Here's how the part is built. I have some questions about the finished solid (model axes, mm). A direction names the side the tool comes from. Give positions to 0.01 mm unless a question says otherwise; leave off trailing zeros. Write each loop counter-clockwise with the first axis right and the second up, starting at its lowest first coordinate (ties: lowest second). Pieces come first, ordered by that corner, then holes. Notation, with made-up numbers: (19, 17) -> (46, 17) arc R25 ccw to (46, 56) -> close; hole circle Ø7 at (-30.5, 79). An arc over 180 degrees is marked (long way). Return JSON: item names as keys, results as strings.
from build123d import *

# Parameters (mm, degrees)
EXTRUDE_1_DEPTH     = 11
SKETCH_2_R          = 2.05
CUT_EXTRUDE_1_DEPTH = 12
SKETCH_3_R          = 3.6
CUT_EXTRUDE_2_DEPTH = 10


with BuildPart() as part:
    # 草图1 → 凸台-拉伸1 (new body)
    with BuildSketch(Plane(origin=(0, 0, 0), x_dir=(1, 0, 0), z_dir=(0, 1, 0))):
        with BuildLine():
            Line((-6, -13), (-6, 13))
            ThreePointArc((-6, 13), (0, 19), (6, 13))
            Line((6, 13), (6, -13))
            ThreePointArc((6, -13), (0, -19), (-6, -13))
        make_face()
    extrude(amount=EXTRUDE_1_DEPTH)

    # 草图2 → 切除-拉伸1 (cut, through all)
    with BuildSketch(Plane(origin=(0, 11, 0), x_dir=(1, 0, 0), z_dir=(0, 1, 0))):
        with Locations((0, 13)):
            Circle(SKETCH_2_R)
        with Locations((0, -13)):
            Circle(SKETCH_2_R)
    extrude(amount=-CUT_EXTRUDE_1_DEPTH, mode=Mode.SUBTRACT)

    # 草图3 → 切除-拉伸2 (cut)
    with BuildSketch(Plane.ZY.offset(6)):
        with Locations((0, 5.5)):
            Circle(SKETCH_3_R)
    extrude(amount=-CUT_EXTRUDE_2_DEPTH, mode=Mode.SUBTRACT)


solid = part.part
1. If I drill on line 1 (Y direction, x = 1.25, z = 0); line 2 (Z direction, x = 0.5, y = 1.75); line 3 (Z direction, x = 0, y = 3.25), over which ranges is the centre line in solid material (lowest first)? Write a range as [from, to].
Taken from the geometry:
{"line 1": "y = [0, 1.9], [9.1, 11]", "line 2": "z = [-18.98, -14.99], [-11.01, 11.01], [14.99, 18.98]", "line 3": "z = [-19, -15.05], [-10.95, -2.81], [2.81, 10.95], [15.05, 19]"}
2. Suppose I cut it at C-C, the plane z = -14. List the corners of the cut face in (x, y) for me.
Taken from the geometry:
{"outline": "(-5.92, 0) -> (-1.79, 0) -> (-1.79, 11) -> (-5.92, 11) -> close; (1.79, 0) -> (5.92, 0) -> (5.92, 11) -> (1.79, 11) -> close"}
3. Suppose I cut it at A-A, the plane x = 0. List the corners of the cut face in (y, z) for me.
Taken from the geometry:
{"outline": "(0, -19) -> (11, -19) -> (11, -15.05) -> (0, -15.05) -> close; (0, -10.95) -> (11, -10.95) -> (11, 10.95) -> (0, 10.95) -> close; (0, 15.05) -> (11, 15.05) -> (11, 19) -> (0, 19) -> close; hole circle Ø7.2 at (5.5, 0)"}
4. Suppose I cut it at D-D, the plane z = 0. List the corners of the cut face in (x, y) for me.
Taken from the geometry:
{"outline": "(-6, 0) -> (6, 0) -> (6, 11) -> (-6, 11) -> (-6, 9.1) -> (4, 9.1) -> (4, 1.9) -> (-6, 1.9) -> close"}
5. Which directions (+Z, -Z, +X, -X, +Y, -Y) give clear straight access to the entire face, cutting with the end or side of a thin tool? Please do faces 1 (the face through (-6, 3, 3)), 2 (the face through (-1.07, 9.07, -0.47)).
Taken from the geometry:
{"face 1": "+Z, -Z, -X, +Y, -Y", "face 2": "-X"}
6. Suppose I cut it at B-B, the plane y = 1. List the corners of the cut face in (x, z) for me, and give its area (3 significant figures).
Taken from the geometry:
{"outline": "(-6, -13) arc R6 ccw to (6, -13) -> (6, 13) arc R6 ccw to (-6, 13) -> close; hole circle Ø4.1 at (0, -13); hole circle Ø4.1 at (0, 13)", "area": "399 mm²"}
7. If we mould it in two halves opening along X, with no side actions, what happens to faces 3 (the face through (6, 5, 0)), 4 (the face through (-0.444, 5.577, 15.001)), 5 (the face through (0, 5, 19))? For each: released by +X, released by -X, zero draft, split by the parting line, or undercut.
Taken from the geometry:
{"face 3": "released by +X", "face 4": "undercut", "face 5": "split by the parting line"}
8. For pin 1 Ø5 at (x, z) = (-0.5, 14) entering from -Y; pin 2 Ø4 at (x, y) = (3, 3) entering from -Z; pin 3 Ø2 at (y, z) = (4, 0.5) entering from -X, each with a flat end and sliding along its axis, tell me the tip position at first contact or that it passes through.
Taken from the geometry:
{"pin 1": "stops at y = 0", "pin 2": "stops at z = -18.92", "pin 3": "stops at x = 4"}
